```python
from build123d import *

# Parameters (mm, degrees)
SKETCH_1_R          = 15.875
SKETCH_1_R_2        = 7.14375
EXTRUDE_1_DEPTH     = 25.4
SKETCH_2_R          = 2
CUT_EXTRUDE_1_DEPTH = 25.4


with BuildPart() as part:
    # 스케치1 → 보스-돌출1 (new body)
    with BuildSketch(Plane(origin=(0, 0, 0), x_dir=(1, 0, 0), z_dir=(0, 1, 0))):
        Circle(SKETCH_1_R)
        Circle(SKETCH_1_R_2, mode=Mode.SUBTRACT)
    extrude(amount=EXTRUDE_1_DEPTH)

    # 스케치2 → 컷-돌출1 (cut)
    with BuildSketch(Plane(origin=(0, 25.4, 0), x_dir=(1, 0, 0), z_dir=(0, 1, 0))):
        with Locations((0, 11.509375)):
            Circle(SKETCH_2_R)
        with Locations((5.7546875, 9.967411132)):
            Circle(SKETCH_2_R)
        with Locations((9.967411132, 5.7546875)):
            Circle(SKETCH_2_R)
        with Locations((11.509375, 0)):
            Circle(SKETCH_2_R)
        with Locations((9.967411132, -5.7546875)):
            Circle(SKETCH_2_R)
        with Locations((5.7546875, -9.967411132)):
            Circle(SKETCH_2_R)
        with Locations((0, -11.509375)):
            Circle(SKETCH_2_R)
        with Locations((-5.7546875, -9.967411132)):
            Circle(SKETCH_2_R)
        with Locations((-9.967411132, -5.7546875)):
            Circle(SKETCH_2_R)
        with Locations((-11.509375, 0)):
            Circle(SKETCH_2_R)
        with Locations((-9.967411132, 5.7546875)):
            Circle(SKETCH_2_R)
        with Locations((-5.7546875, 9.967411132)):
            Circle(SKETCH_2_R)
    extrude(amount=-CUT_EXTRUDE_1_DEPTH, mode=Mode.SUBTRACT)


solid = part.part
```
Work out the finished part from the listing and answer in its coordinate system (mm). Give positions to 0.01 mm unless a question says otherwise; leave off trailing zeros. Loops run counter-clockwise (first coordinate to the right, second up) from the corner with the lowest first, then second, coordinate; pieces in that order, holes last. Notation, with made-up numbers: (24, 19.25) -> (44, 19.25) arc R17 ccw to (44, 38.25) -> close; hole circle Ø11 at (44, -33.75). An arc over 180 degrees is marked (long way). Write item = value, one per line. Start each with the question number.
(1) The mould has two halves that part along Z. Classify faces 1 (the cylindrical face through (13.357, 12.878, 0.766)), 2 (the cylindrical face through (-3.441, 12.522, 15.497)), 3 (the flat face through (7, 0, 3)), 4 (the cylindrical face through (-13.507, 12.878, -0.088)): +Z half, -Z half, draft (parallel to the pull), parting line (faces both ways), or undercut.
(2) Given pin 1 Ø3 at (x, z) = (0, 11.51) entering from -Y; pin 2 Ø2 at (x, y) = (-1.5, 20) entering from +Z; pin 3 Ø3 at (x, y) = (5, 16.5) entering from -Z; pin 4 Ø5 at (x, y) = (5, 10.5) entering from +Z, each flat-ended and moving along its own axis, determine where each tip first touches the part or whether it passes through.
(3) Find section C-C on x = -13. Give the vertices of the cut face in (y, z), and give its area (3 significant figures).
(4) Find section B-B on z = 0. Give the vertices of the cut face in (x, y) (3 decimals), and give its area (3 significant figures).
(5) Find the intervals of material crossed by probe 1 along Z at (x, y) = (0, 8.75) (3 decimals); probe 2 along X at (y, z) = (6.5, 11), in increasing order. Write a range as from..to.
(6) Find section D-D on y = 4.75. Give the number of separate pieces and of enclosed holes in the cut face, and give its area (3 significant figures).
(7) Find section A-A on x = 0. Give the vertices of the cut face in (y, z) (3 decimals), and give its area (3 significant figures).
From the geometry:
q1.face_1 = undercut
q1.face_2 = parting line
q1.face_3 = draft
q1.face_4 = undercut
q2.pin_1 = through
q2.pin_2 = 15.87
q2.pin_3 = -15.48
q2.pin_4 = 15.68
q3.outline = (0, -9.11) -> (25.4, -9.11) -> (25.4, -1.33) -> (0, -1.33) -> close; (0, 1.33) -> (25.4, 1.33) -> (25.4, 9.11) -> (0, 9.11) -> close
q3.area = 395 mm^2
q4.outline = (-15.875, 0) -> (-13.509, 0) -> (-13.509, 25.4) -> (-15.875, 25.4) -> close; (-9.509, 0) -> (-7.144, 0) -> (-7.144, 25.4) -> (-9.509, 25.4) -> close; (7.144, 0) -> (9.509, 0) -> (9.509, 25.4) -> (7.144, 25.4) -> close; (13.509, 0) -> (15.875, 0) -> (15.875, 25.4) -> (13.509, 25.4) -> close
q4.area = 240 mm^2
q5.probe_1 = -15.875..-13.509, -9.509..-7.144, 7.144..9.509, 13.509..15.875
q5.probe_2 = -11.45..-7.47, -4.04..-1.93, 1.93..4.04, 7.47..11.45
q6.separate_pieces = 1
q6.enclosed_holes = 13
q6.area = 481 mm^2
q7.outline = (0, -15.875) -> (25.4, -15.875) -> (25.4, -13.509) -> (0, -13.509) -> close; (0, -9.509) -> (25.4, -9.509) -> (25.4, -7.144) -> (0, -7.144) -> close; (0, 7.144) -> (25.4, 7.144) -> (25.4, 9.509) -> (0, 9.509) -> close; (0, 13.509) -> (25.4, 13.509) -> (25.4, 15.875) -> (0, 15.875) -> close
q7.area = 240 mm^2
